Source: CAD feature listing. Evaluate the final solid. Frame: model axes, mm. A direction names the side the tool comes from. Coordinates: 2 decimals unless noted, no trailing zeros. Order: outer loops, then holes, each group sorted by start corner. A loop starts at its lowest first (then second) coordinate and runs counter-clockwise, first axis right, second up. Notation, with made-up numbers: (27, 47.5) -> (81, 47.5) arc R9 ccw to (81, 52.5) -> close; hole circle Ø2 at (54, -38.5). An arc over 180 degrees is marked (long way). Write each question's results on one line, items separated by ' | '. Start each with the question number.
from build123d import *


with BuildPart() as part:
    # Sketch1 → Revolve1 (revolve)
    with BuildSketch(Plane.XY, mode=Mode.PRIVATE) as revolve1_sk:
        with BuildLine():
            Line((0, 1.5), (0, 3.5))
            Line((0, 3.5), (-4, 3.5))
            Line((-4, 3.5), (-4, 8.4))
            Line((-4, 8.4), (0, 8.4))
            Line((0, 8.4), (0, 10))
            ThreePointArc((0, 10), (-0.732233047, 11.767766953), (-2.5, 12.5))
            Line((-2.5, 12.5), (-10.5, 12.5))
            ThreePointArc((-10.5, 12.5), (-12.267766953, 11.767766953), (-13, 10))
            Line((-13, 10), (-13, 8.4))
            Line((-13, 8.4), (-9, 8.4))
            Line((-9, 8.4), (-9, 3.5))
            Line((-9, 3.5), (-13, 3.5))
            Line((-13, 3.5), (-13, 1.5))
            Line((-13, 1.5), (0, 1.5))
        make_face()
    revolve(revolve1_sk.sketch.rotate(Axis((-1000.574907176, 0, 0), (1, 0, 0)), 90), axis=Axis((-1000.574907176, 0, 0), (1, 0, 0)))


solid = part.part
(1) Section C-C on x = -3.5. Return the cut outline in (y, z).
(2) First-contact query: P1, Ø1.5, axis at x = -11.5, z = -2, coming from the +Y side; P2, Ø2, axis at x = -5.5, y = -5.5, coming from the +Z side; P3, Ø2, axis at y = -2.5, z = 4, coming from the +X side; P4, Ø2.5, axis at y = 0, z = 0, coming from the +X side. Flat tips, straight axial feed; report the tip coordinate or a pass-through.
(3) Draft query along Z for faces 1 (the cylindrical face through (-10.972, -2.523, 8.012)), 2 (the flat face through (-13, -7, -5)), 3 (the flat face through (-4, 0, -4)), 4 (the cylindrical face through (-6.556, -3.755, 11.923)). Return one class per face: released by +Z, released by -Z, zero draft, split by the parting line, or undercut.
(4) Section D-D on x = -5.75. Return the cut outline in (y, z), then the cut area to 3 significant figures.
(5) Section A-A on z = 0. Return the cut outline in (x, y), then the cut area to 3 significant figures.
(6) Line query: L1, parallel to Z at x = -2.75, y = -2; L2, parallel to Y at x = -10.7, z = 0; L3, parallel to Y at x = -5.5, z = 0. Output: solid intervals per line, ascending.
(7) Reachability of faces 5 (the flat face through (0, -7, 5)), 6 (the cylindrical face through (-2.028, 3.105, 1.615)), 7 (the cylindrical face through (-11.028, 3.105, 1.615)) from +Z, -Z, +X, -X, +Y, -Y: full face, straight path, thin tool, end or side. Return the list, or none.
Results list:
1) outline: circle Ø25 at (0, 0); circle Ø7 at (0, 0); hole circle Ø16.8 at (0, 0); hole circle Ø3 at (0, 0)
2) P1: stops at y = 12.37 | P2: stops at z = 11.66 | P3: stops at x = -4 | P4: passes through
3) face 1: undercut | face 2: zero draft | face 3: undercut | face 4: split by the parting line
4) outline: circle Ø25 at (0, 0); hole circle Ø3 at (0, 0) | area: 484 mm²
5) outline: (-13, -10) arc R2.5 ccw to (-10.5, -12.5) -> (-2.5, -12.5) arc R2.5 ccw to (0, -10) -> (0, -8.4) -> (-4, -8.4) -> (-4, -3.5) -> (0, -3.5) -> (0, -1.5) -> (-13, -1.5) -> (-13, -3.5) -> (-9, -3.5) -> (-9, -8.4) -> (-13, -8.4) -> close; (-13, 1.5) -> (0, 1.5) -> (0, 3.5) -> (-4, 3.5) -> (-4, 8.4) -> (0, 8.4) -> (0, 10) arc R2.5 ccw to (-2.5, 12.5) -> (-10.5, 12.5) arc R2.5 ccw to (-13, 10) -> (-13, 8.4) -> (-9, 8.4) -> (-9, 3.5) -> (-13, 3.5) -> close | area: 202 mm²
6) L1: z = -12.34 to -8.16, -2.87 to 2.87, 8.16 to 12.34 | L2: y = -12.49 to -8.4, -3.5 to -1.5, 1.5 to 3.5, 8.4 to 12.49 | L3: y = -12.5 to -1.5, 1.5 to 12.5
7) face 5: +Z, -Z, +X, +Y, -Y | face 6: +X | face 7: -X
